```python
from build123d import *

# Parameters (mm, degrees)
SKETCH_1_R          = 13
EXTRUDE_1_DEPTH     = 7
SKETCH_2_R          = 12
CUT_EXTRUDE_1_DEPTH = 3
EXTRUDE_2_DEPTH     = 7


with BuildPart() as part:
    # 草图1 → 凸台-拉伸1 (new body)
    with BuildSketch(Plane(origin=(0, 0, 0), x_dir=(1, 0, 0), z_dir=(0, 1, 0))):
        with Locations(Location((0, 0, 0), (0, 0, 270))):
            Circle(SKETCH_1_R)
    extrude(amount=EXTRUDE_1_DEPTH)

    # 草图2 → 切除-拉伸1 (cut)
    with BuildSketch(Plane(origin=(0, 7, 0), x_dir=(1, 0, 0), z_dir=(0, 1, 0))):
        with Locations(Location((0, 0, 0), (0, 0, 270))):
            Circle(SKETCH_2_R)
    extrude(amount=-CUT_EXTRUDE_1_DEPTH, mode=Mode.SUBTRACT)

    # 草图3 → 凸台-拉伸2 (add, through all)
    with BuildSketch(Plane(origin=(0, 7, 0), x_dir=(1, 0, 0), z_dir=(0, 1, 0))):
        Polygon((-12.123665589, 4.692199131), (-11.044603538, 4.692199131), (-11.653830585, 5.760922904), (-12.732892635, 5.760922904), align=None)
        Polygon((-11.124688039, 6.726166519), (-10.062019365, 6.53878936), (-10.476408948, 7.697067984), (-11.539077622, 7.884445143), align=None)
        Polygon((-9.787692472, 8.555762741), (-8.773705825, 8.186701784), (-8.980666927, 9.399341549), (-9.994653573, 9.768402506), align=None)
        Polygon((-8.153302822, 10.125396442), (-7.218807673, 9.585865416), (-7.212051886, 10.816020876), (-8.146547034, 11.355551902), align=None)
        Polygon((-6.271179191, 11.387375095), (-5.444569703, 10.693767379), (-5.224302297, 11.904060883), (-6.050911785, 12.597668599), align=None)
        Polygon((-4.198508954, 12.303354118), (-3.504901238, 11.47674463), (-3.077814927, 12.630402023), (-3.771422644, 13.457011511), align=None)
        Polygon((-1.998269147, 12.845501953), (-1.458738122, 11.911006804), (-0.837809708, 12.97297479), (-1.377340734, 13.907469938), align=None)
        Polygon((0.262687056, 12.99734571), (0.631748014, 11.983359064), (1.427651935, 12.921370282), (1.058590978, 13.935356928), align=None)
        Polygon((2.515661647, 12.754271695), (2.703038805, 11.691603022), (3.649735097, 12.477156476), (3.462357938, 13.53982515), align=None)
        Polygon((4.692199131, 12.123665589), (4.692199131, 11.044603538), (5.760922904, 11.653830585), (5.760922904, 12.732892635), align=None)
        Polygon((6.726166519, 11.124688039), (6.53878936, 10.062019365), (7.697067984, 10.476408948), (7.884445143, 11.539077622), align=None)
        Polygon((8.555762741, 9.787692472), (8.186701784, 8.773705825), (9.399341549, 8.980666927), (9.768402506, 9.994653573), align=None)
        Polygon((10.125396442, 8.153302822), (9.585865416, 7.218807673), (10.816020876, 7.212051886), (11.355551902, 8.146547034), align=None)
        Polygon((11.387375095, 6.271179191), (10.693767379, 5.444569703), (11.904060883, 5.224302297), (12.597668599, 6.050911785), align=None)
        Polygon((12.303354118, 4.198508954), (11.47674463, 3.504901238), (12.630402023, 3.077814927), (13.457011511, 3.771422644), align=None)
        Polygon((12.845501953, 1.998269147), (11.911006804, 1.458738122), (12.97297479, 0.837809708), (13.907469938, 1.377340734), align=None)
        Polygon((12.99734571, -0.262687056), (11.983359064, -0.631748014), (12.921370282, -1.427651935), (13.935356928, -1.058590978), align=None)
        Polygon((12.754271695, -2.515661647), (11.691603022, -2.703038805), (12.477156476, -3.649735097), (13.53982515, -3.462357938), align=None)
        Polygon((12.123665589, -4.692199131), (11.044603538, -4.692199131), (11.653830585, -5.760922904), (12.732892635, -5.760922904), align=None)
        Polygon((11.124688039, -6.726166519), (10.062019365, -6.53878936), (10.476408948, -7.697067984), (11.539077622, -7.884445143), align=None)
        Polygon((9.787692472, -8.555762741), (8.773705825, -8.186701784), (8.980666927, -9.399341549), (9.994653573, -9.768402506), align=None)
        Polygon((8.153302822, -10.125396442), (7.218807673, -9.585865416), (7.212051886, -10.816020876), (8.146547034, -11.355551902), align=None)
        Polygon((6.271179191, -11.387375095), (5.444569703, -10.693767379), (5.224302297, -11.904060883), (6.050911785, -12.597668599), align=None)
        Polygon((4.198508954, -12.303354118), (3.504901238, -11.47674463), (3.077814927, -12.630402023), (3.771422644, -13.457011511), align=None)
        Polygon((1.998269147, -12.845501953), (1.458738122, -11.911006804), (0.837809708, -12.97297479), (1.377340734, -13.907469938), align=None)
        Polygon((-0.262687056, -12.99734571), (-0.631748014, -11.983359064), (-1.427651935, -12.921370282), (-1.058590978, -13.935356928), align=None)
        Polygon((-2.515661647, -12.754271695), (-2.703038805, -11.691603022), (-3.649735097, -12.477156476), (-3.462357938, -13.53982515), align=None)
        Polygon((-4.692199131, -12.123665589), (-4.692199131, -11.044603538), (-5.760922904, -11.653830585), (-5.760922904, -12.732892635), align=None)
        Polygon((-6.726166519, -11.124688039), (-6.53878936, -10.062019365), (-7.697067984, -10.476408948), (-7.884445143, -11.539077622), align=None)
        Polygon((-8.555762741, -9.787692472), (-8.186701784, -8.773705825), (-9.399341549, -8.980666927), (-9.768402506, -9.994653573), align=None)
        Polygon((-10.125396442, -8.153302822), (-9.585865416, -7.218807673), (-10.816020876, -7.212051886), (-11.355551902, -8.146547034), align=None)
        Polygon((-11.387375095, -6.271179191), (-10.693767379, -5.444569703), (-11.904060883, -5.224302297), (-12.597668599, -6.050911785), align=None)
        Polygon((-12.303354118, -4.198508954), (-11.47674463, -3.504901238), (-12.630402023, -3.077814927), (-13.457011511, -3.771422644), align=None)
        Polygon((-12.845501953, -1.998269147), (-11.911006804, -1.458738122), (-12.97297479, -0.837809708), (-13.907469938, -1.377340734), align=None)
        Polygon((-12.99734571, 0.262687056), (-11.983359064, 0.631748014), (-12.921370282, 1.427651935), (-13.935356928, 1.058590978), align=None)
        Polygon((-12.754271695, 2.515661647), (-11.691603022, 2.703038805), (-12.477156476, 3.649735097), (-13.53982515, 3.462357938), align=None)
    extrude(amount=-EXTRUDE_2_DEPTH)


solid = part.part
```
Check sheet for the modelled part. Datum: model origin and axes. Units: mm. A direction names the side the tool comes from. Round coordinates to 2 decimals unless told otherwise and drop trailing zeros. Answer as a JSON object with one key per item and string values. Group by question number.
Q1. Scan lines: line 1 along Z through (x, y) = (0, 5.9); line 2 along Y through (x, z) = (-7.25, 9.25). Record each from-to range of solid material in increasing order. Write a range as [from, to].
Q2. Gauge pin test, flat ends, axial feed: P1, Ø2, axis at y = 6, z = 6, coming from the -X side; P2, Ø4, axis at y = 4.5, z = -9, coming from the -X side; P3, Ø1.2, axis at y = 5, z = 12.5, coming from the -X side. Record the tip position at first contact, or that the pin passes through.
Q3. Set-up check for faces 5 (the face through (-6.741, 3.451, -11.116)), 6 (the face through (1.683, 3.549, 13.384)), 7 (the face through (-12.246, 3.549, 5.632)), 8 (the face through (-12, 4, -5.761)): record each of +Z, -Z, +X, -X, +Y, -Y from which the full face is reachable in a straight line by a thin tool's end or side.
Q4. Mould release check, pull along X, two halves, no side actions. Record for faces 1 (the face through (-1.98, 3.45, 12.85)), 2 (the face through (1.98, 3.45, -12.85)), 3 (the face through (-9.58, 3.55, 9.48)), 4 (the face through (12.75, 3.45, -2.53)): released by +X, released by -X, zero draft, split by the parting line, or undercut.
Solution:
{
 "1": {"line 1": "z = [-13, -12], [12, 13]", "line 2": "y = [0, 4]"},
 "2": {"P1": "stops at x = -12.6", "P2": "stops at x = -11.54", "P3": "stops at x = -5.76"},
 "3": {"face 5": "-Z, +Y, -Y", "face 6": "+Z, +Y, -Y", "face 7": "-X, +Y, -Y", "face 8": "-Z, -X, +Y, -Y"},
 "4": {"face 1": "undercut", "face 2": "undercut", "face 3": "released by -X", "face 4": "released by +X"}
}
